Solid Edge part; units mm, degrees
sketch "Sketch1" plane through (0, 0, 0) normal (0, 0, 1) x (1, 0, 0)
  circle A0 centre (0, 0) radius 5
  line L0 (169.7056, -5) -> (221.7311, -5)
  arc A1 (221.7311, -5) -> (158.8762, -151.8052) centre (270.199, -112.6099) ccw
  line L1 (123.5355, -116.4645) -> (158.8762, -151.8052)
  arc A2 (116.4645, -123.5355) -> (123.5355, -116.4645) centre (120, -120) cw
  line L2 (116.4645, -123.5355) -> (153.252, -160.3231)
  arc A3 (153.252, -160.3231) -> (5, -219.6849) centre (111.4323, -270.6868) ccw
  line L3 (5, -169.7056) -> (5, -219.6849)
  arc A4 (-5, -169.7056) -> (5, -169.7056) centre (0, -169.7056) cw
  line L4 (-5, -169.7056) -> (-5, -221.7311)
  arc A5 (-5, -221.7311) -> (-151.8052, -158.8762) centre (-112.6099, -270.199) ccw
  line L5 (-116.4645, -123.5355) -> (-151.8052, -158.8762)
  arc A6 (-123.5355, -116.4645) -> (-116.4645, -123.5355) centre (-120, -120) cw
  line L6 (-123.5355, -116.4645) -> (-160.3231, -153.252)
  arc A7 (-160.3231, -153.252) -> (-219.6849, -5) centre (-270.6868, -111.4323) ccw
  line L7 (-169.7056, -5) -> (-219.6849, -5)
  arc A8 (-169.7056, 5) -> (-169.7056, -5) centre (-169.7056, 0) cw
  line L8 (-169.7056, 5) -> (-221.7311, 5)
  arc A9 (-221.7311, 5) -> (-158.8762, 151.8052) centre (-270.199, 112.6099) ccw
  line L9 (-123.5355, 116.4645) -> (-158.8762, 151.8052)
  arc A10 (-116.4645, 123.5355) -> (-123.5355, 116.4645) centre (-120, 120) cw
  line L10 (-116.4645, 123.5355) -> (-153.252, 160.3231)
  arc A11 (-153.252, 160.3231) -> (-5, 219.6849) centre (-111.4323, 270.6868) ccw
  line L11 (-5, 169.7056) -> (-5, 219.6849)
  arc A12 (5, 169.7056) -> (-5, 169.7056) centre (0, 169.7056) cw
  line L12 (5, 169.7056) -> (5, 221.7311)
  arc A13 (5, 221.7311) -> (151.8052, 158.8762) centre (112.6099, 270.199) ccw
  line L13 (116.4645, 123.5355) -> (151.8052, 158.8762)
  arc A14 (123.5355, 116.4645) -> (116.4645, 123.5355) centre (120, 120) cw
  line L14 (123.5355, 116.4645) -> (160.3231, 153.252)
  arc A15 (160.3231, 153.252) -> (219.6849, 5) centre (270.6868, 111.4323) ccw
  line L15 (169.7056, 5) -> (219.6849, 5)
  arc A16 (169.7056, -5) -> (169.7056, 5) centre (169.7056, 0) cw
extrude "Protrusion1" add sketch "Sketch1" along normal blind 10
Geometry: final body of the model. Coordinates: model frame, mm. A direction names the side the tool comes from. Round coordinates to 2 decimals unless told otherwise and drop trailing zeros. Order: outer loops, then holes, each group sorted by start corner. A loop starts at its lowest first (then second) coordinate and runs counter-clockwise, first axis right, second up. Notation, with made-up numbers: (-37, 13) -> (-23, 13) arc R10 cw to (-23, 17) -> close; hole circle Ø5 at (55.25, 45.5). An arc over 180 degrees is marked (long way). Use one line per item in the form item = value. Start each with the question number.
1. Reachability of faces 1 (the face through (-5, 194, 5)), 2 (the face through (195, -5, 5)), 3 (the face through (133.89, 140.96, 4.93)), 4 (the face through (-164.707, 0.11, 4.93)), 5 (the face through (-5, -195, 5)) from +Z, -Z, +X, -X, +Y, -Y: full face, straight path, thin tool, end or side. Return the list, or none.
2. Cut plane C-C (x = -98). Return the cut outline in (y, z), then the cut area to 3 significant figures.
3. Line query: probe 1 along Y at (x, z) = (0, 5); probe 2 along X at (y, z) = (122, 1.5); probe 3 along X at (y, z) = (113.5, 1). Output: solid intervals per line, ascending.
4. Cut plane D-D (y = 88). Return the cut outline in (x, z), then the cut area to 3 significant figures.
5. Pin query (flat end, axial travel): pin 1 Ø3 at (x, z) = (-206, 5.5) entering from +Y; pin 2 Ø1 at (y, z) = (123.5, 6) entering from +X; pin 3 Ø6 at (y, z) = (-177.5, 2.5) entering from +X. Return the tip coordinate at first contact, or that it passes through.
6. Cut plane B-B (y = -131.5). Return the cut outline in (x, z), then the cut area to 3 significant figures.
7. Draft query along Y for faces 6 (the face through (-194, -5, 5)), 7 (the face through (5, -194, 5)), 8 (the face through (-66.424, 161.585, 4.93)), 9 (the face through (-141.67, -134.6, 4.93)). Return one class per face: pulls with the +Y half, pulls with the -Y half, needs draft (parallel to the pull), parting line crosses it, or undercut.
Solution:
q1.face_1 = +Z, -Z, +Y
q1.face_2 = +Z, -Z, +X
q1.face_3 = +Z, -Z
q1.face_4 = +Z, -Z, -X
q1.face_5 = +Z, -Z, -Y
q2.outline = (-153.09, 0) -> (153.43, 0) -> (153.43, 10) -> (-153.09, 10) -> close
q2.area = 3,070 mm^2
q3.probe_1 = -164.71 to -5, 5 to 164.71
q3.probe_2 = -152.55 to -129.07, -115.42 to 115.42, 129.07 to 153.14
q3.probe_3 = -152.18 to 152.68
q4.outline = (-154.77, 0) -> (155.02, 0) -> (155.02, 10) -> (-154.77, 10) -> close
q4.area = 3,100 mm^2
q5.pin_1 = 14.57
q5.pin_2 = 153.34
q5.pin_3 = 43.04
q6.outline = (-154.38, 0) -> (-138.57, 0) -> (-138.57, 10) -> (-154.38, 10) -> close; (-124.43, 0) -> (124.43, 0) -> (124.43, 10) -> (-124.43, 10) -> close; (138.57, 0) -> (153.7, 0) -> (153.7, 10) -> (138.57, 10) -> close
q6.area = 2,800 mm^2
q7.face_6 = undercut
q7.face_7 = needs draft
q7.face_8 = pulls with the +Y half
q7.face_9 = undercut
